Build history of the part. All positions in model axes, mm. Face numbers are marked on the shaded views. Round coordinates to 2 decimals unless told otherwise and drop trailing zeros. Write each loop counter-clockwise with the first axis right and the second up, starting at its lowest first coordinate (ties: lowest second). Pieces come first, ordered by that corner, then holes.
1) Saw through at B-B (y = 7.5). Write the cut outline in (x, z).
2) Saw through at A-A (y = 10). Write the cut outline in (x, z).
3) Saw through at C-C (z = 17.5). Write the cut outline in (x, y), plus the area to 3 significant figures.
4) Flat gauge pins, fed straight in: pin 1 (1.2 mm diameter, centred on x = 18, z = 17.5, fed in from -Y); pin 2 (1 mm diameter, centred on y = 10.5, z = 1, fed in from +X). Where does each tip first touch, or does it go through?
5) Saw through at D-D (x = -11.5). Write the cut outline in (y, z), plus the area to 3 significant figures.
6) Wall check: probe 1 along X at (y, z) = (6.25, -17.5); probe 2 along X at (y, z) = (14.25, -17.5); probe 3 along Z at (x, y) = (18, 6). Give the ranges that are in metal, low to high.
7) Pull direction Z, two halves, no side cores. Call the marked faces 1, 2 and 3: +Z half, -Z half, draft (parallel to the pull), parting line (faces both ways), or undercut.
from build123d import *

# Parameters (mm, degrees)
BOSS_EXTRUDE1_DEPTH     = 25
CUT_EXTRUDE1_DEPTH      = 38.423121195
CUT_EXTRUDE1_DEPTH_BACK = 38.423121195
SKETCH2_R               = 12.8
SKETCH3_R               = 2
CUT_EXTRUDE2_DEPTH      = 7.5
SKETCH4_R               = 2
CUT_EXTRUDE3_DEPTH      = 7.5


with BuildPart() as part:
    # Sketch1 → Boss-Extrude1 (new, symmetric)
    with BuildSketch(Plane(origin=(0, 0, 0), x_dir=(0, 0, -1), z_dir=(1, 0, 0))):
        with BuildLine():
            Line((-19, 0.6), (19, 0.6))
            ThreePointArc((19, 0.6), (21.828427125, 1.771572875), (23, 4.6))
            Line((23, 4.6), (23, 11.7))
            ThreePointArc((23, 11.7), (21.828427125, 14.528427125), (19, 15.7))
            Line((19, 15.7), (-19, 15.7))
            ThreePointArc((-19, 15.7), (-21.828427125, 14.528427125), (-23, 11.7))
            Line((-23, 11.7), (-23, 4.6))
            ThreePointArc((-23, 4.6), (-21.828427125, 1.771572875), (-19, 0.6))
        make_face()
    extrude(amount=BOSS_EXTRUDE1_DEPTH, both=True)

    # Sketch2 → Cut-Extrude1 (cut, two sides: drawn at the far end of the back side and taken through both)
    with BuildSketch(Plane(origin=(0, 0, 0), x_dir=(0, 0, -1), z_dir=(1, 0, 0)).offset(-CUT_EXTRUDE1_DEPTH_BACK)):
        Circle(SKETCH2_R)
    extrude(amount=CUT_EXTRUDE1_DEPTH + CUT_EXTRUDE1_DEPTH_BACK, mode=Mode.SUBTRACT)

    # Sketch3 → Cut-Extrude2 (cut)
    with BuildSketch(Plane(origin=(0, 0.6, 0), x_dir=(1, 0, 0), z_dir=(0, 1, 0))):
        with Locations(Location((18, -17.5, 0), (0, 0, 228.590377891))):
            Circle(SKETCH3_R)
        with Locations(Location((18, 17.5, 0), (0, 0, 48.590377891))):
            Circle(SKETCH3_R)
        with Locations(Location((-18, -17.5, 0), (0, 0, 228.590377891))):
            Circle(SKETCH3_R)
        with Locations(Location((-18, 17.5, 0), (0, 0, 48.590377891))):
            Circle(SKETCH3_R)
    extrude(amount=CUT_EXTRUDE2_DEPTH, mode=Mode.SUBTRACT)

    # Sketch4 → Cut-Extrude3 (cut)
    with BuildSketch(Plane(origin=(0, 15.7, 0), x_dir=(1, 0, 0), z_dir=(0, 1, 0))):
        with Locations(Location((0, -17.5, 0), (0, 0, 270))):
            Circle(SKETCH4_R)
        with Locations(Location((0, 17.5, 0), (0, 0, 270))):
            Circle(SKETCH4_R)
    extrude(amount=-CUT_EXTRUDE3_DEPTH, mode=Mode.SUBTRACT)


solid = part.part
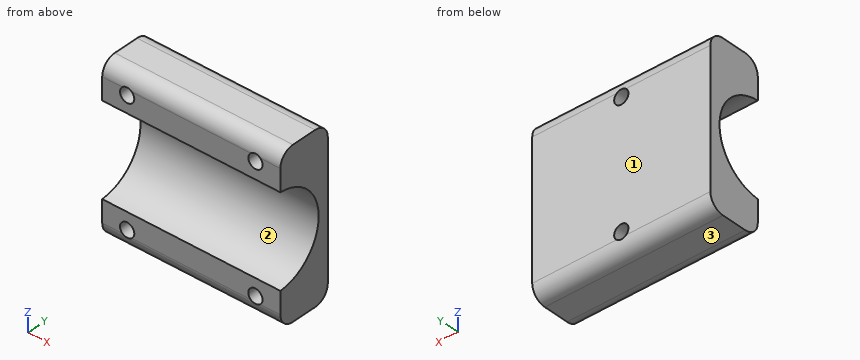
Evaluation:
1. outline: (-25, -23) - (25, -23) - (25, -10.37) - (-25, -10.37) - close; (-25, 10.37) - (25, 10.37) - (25, 23) - (-25, 23) - close; hole circle Ø4 at (-18, -17.5); hole circle Ø4 at (-18, 17.5); hole circle Ø4 at (18, -17.5); hole circle Ø4 at (18, 17.5)
2. outline: (-25, -23) - (25, -23) - (25, -7.99) - (-25, -7.99) - close; (-25, 7.99) - (25, 7.99) - (25, 23) - (-25, 23) - close; hole circle Ø4 at (0, -17.5); hole circle Ø4 at (0, 17.5)
3. outline: (-25, 0.6) - (-20, 0.6) - (-20, 8.1) - (-16, 8.1) - (-16, 0.6) - (16, 0.6) - (16, 8.1) - (20, 8.1) - (20, 0.6) - (25, 0.6) - (25, 15.7) - (2, 15.7) - (2, 8.2) - (-2, 8.2) - (-2, 15.7) - (-25, 15.7) - close
3. area: 665 mm2
4. pin 1: stops at y = 8.1
4. pin 2: passes through
5. outline: (0.6, -19) arc R4 ccw to (4.6, -23) - (11.7, -23) arc R4 ccw to (15.7, -19) - (15.7, 19) arc R4 ccw to (11.7, 23) - (4.6, 23) arc R4 ccw to (0.6, 19) - (0.6, 12.79) arc R12.8 cw to (0.6, -12.79) - close
5. area: 439 mm2
6. probe 1: x = -25 to -20, -16 to 16, 20 to 25
6. probe 2: x = -25 to -2, 2 to 25
6. probe 3: z = -23 to -19.5, -15.5 to -11.31, 11.31 to 15.5, 19.5 to 23
7. face 1: draft
7. face 2: undercut
7. face 3: -Z half
